Could you check a few things on this drawing? It's one solid part, dimensions in mm from its lowest x, y, z. Give positions to 0.01 mm unless a question says otherwise; leave off trailing zeros. Loops run counter-clockwise (first coordinate to the right, second up) from the corner with the lowest first, then second, coordinate; pieces in that order, holes last. Notation, with made-up numbers: (-39.75, 12) - (-14.75, 12) arc R16 ccw to (-14.75, 36) - close; hole circle Ø7 at (78.5, 12). An arc over 180 degrees is marked (long way). Write item = value, one per line.
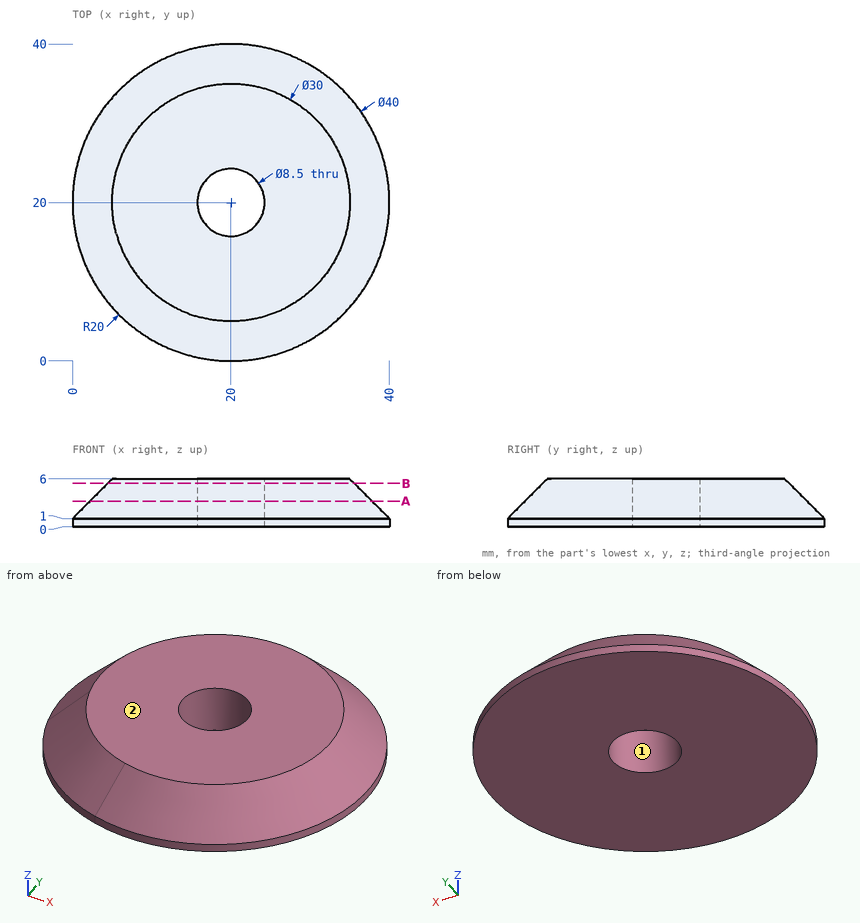
Q1. Imagine slicing it at B-B, the plane z = 5.45. Write out the boundary of the cut face in (x, y).
Output:
outline = (4.99, 15.93) arc R15.55 ccw to (15.93, 4.99) arc R15.55 ccw (long way) to start; hole circle Ø8.5 at (20, 20)
Q2. I need wall thicknesses on L1, parallel to X at y = 23, z = 0.95; L2, parallel to Y at x = 21, z = 3.05; L3, parallel to Y at x = 22.5, z = 2.35. Which ranges of each line are inside material? Lowest first, please.
Output:
L1 = 0.23 to 16.99, 23.01 to 39.77
L2 = 2.08 to 15.87, 24.13 to 37.92
L3 = 1.52 to 16.56, 23.44 to 38.48
Q3. For pin 1 (1 mm diameter, centred on y = 30, z = 3, fed in from -X), with a flat end and sliding along its axis, tell me the tip position at first contact or that it passes through.
Output:
pin_1 = 4.36
Q4. Imagine slicing it at A-A, the plane z = 3.2. Write out the boundary of the cut face in (x, y), then the cut area to 3 significant figures.
Output:
outline = (2.82, 15.35) arc R17.8 ccw to (15.35, 2.82) arc R17.8 ccw (long way) to start; hole circle Ø8.5 at (20, 20)
area = 939 mm2
Q5. We'd pull the mould along X, two halves only. Please class the marked faces 1 and 2: released by +X, released by -X, zero draft, split by the parting line, or undercut.
Output:
face_1 = undercut
face_2 = zero draft
